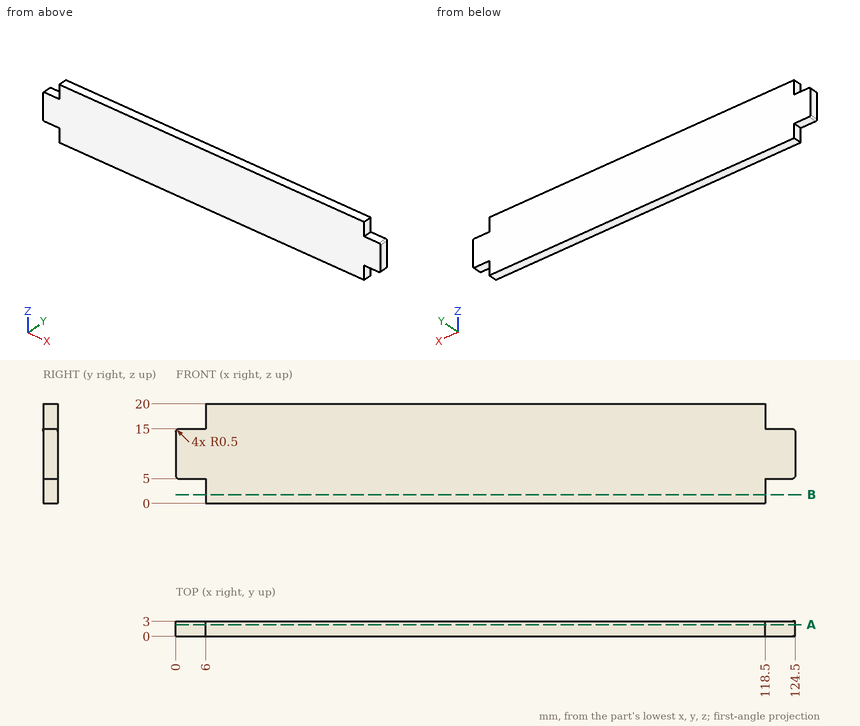
For this review, use the dimensioned drawing (mm, ordinates from the lowest corner) and the shaded views. Coordinates: 2 decimals unless noted, no trailing zeros. Loops run counter-clockwise (first coordinate to the right, second up) from the corner with the lowest first, then second, coordinate; pieces in that order, holes last. Notation, with made-up numbers: (-11.75, 41) - (15.25, 41) arc R22 cw to (15.25, 57) - close; hole circle Ø7 at (-30, 50). An arc over 180 degrees is marked (long way). Use CSV: the item, a comma, the result in double quotes. Start each with the question number.
1) Consider section A-A on y = 2.35. Write out the cut boundary in (x, z).
2) For pin 1 Ø4 at (x, z) = (66, 8.5) entering from -Y; pin 2 Ø1.5 at (x, y) = (122.5, 2) entering from -Z, all flat-tipped, find the tip position at first contact; note any pin that passes through.
3) Consider section B-B on z = 1.75. Write out the cut boundary in (x, y), then the cut area to 4 significant figures.
4) Wall thickness on L1, parallel to X at y = 0.5, z = 17; L2, parallel to X at y = 2.5, z = 5.25: over which ranges is each line inside the solid? List them lowest first. Write a range as from..to.
Geometry says:
1,outline,"(0, 5.5) arc R0.5 ccw to (0.5, 5) - (6, 5) - (6, 0) - (118.5, 0) - (118.5, 5) - (124, 5) arc R0.5 ccw to (124.5, 5.5) - (124.5, 14.5) arc R0.5 ccw to (124, 15) - (118.5, 15) - (118.5, 20) - (6, 20) - (6, 15) - (0.5, 15) arc R0.5 ccw to (0, 14.5) - close"
2,pin 1,"y = 0"
2,pin 2,"z = 5"
3,outline,"(6, 0) - (118.5, 0) - (118.5, 3) - (6, 3) - close"
3,area,"337.5 mm^2"
4,L1,"6..118.5"
4,L2,"0.07..124.43"
